Check sheet for the drawn part. Datum: minimum x, y, z corner. Units: mm. A direction names the side the tool comes from. Coordinates: 2 decimals unless noted, no trailing zeros. Order: outer loops, then holes, each group sorted by start corner. A loop starts at its lowest first (then second) coordinate and runs counter-clockwise, first axis right, second up.
Q1. Set-up check for the marked faces 1 and 2: record each of +Z, -Z, +X, -X, +Y, -Y from which the full face is reachable in a straight line by a thin tool's end or side.
Q2. Depth check by flat-ended pin: P1, Ø5, axis at x = 12.5, y = 13.5, coming from the +Z side; P2, Ø2, axis at x = 21, z = 3.5, coming from the +Y side; P3, Ø2, axis at y = 20, z = 11.5, coming from the -X side; P4, Ø5, axis at x = 8, z = 11, coming from the +Y side. Enter the tip coordinate at first touch or a pass-through.
Q3. Cross-section at B-B, the plane z = 7. Record the boundary of the cut face in (x, y), and give its area (3 significant figures).
Q4. Cross-section at A-A, the plane z = 17.75. Record the boundary of the cut face in (x, y), and give its area (3 significant figures).
Q5. Thickness scan on line 1 (X direction, y = 14, z = 17.25); line 2 (X direction, y = 26.5, z = 3). Record the ranges inside material, lowest first.
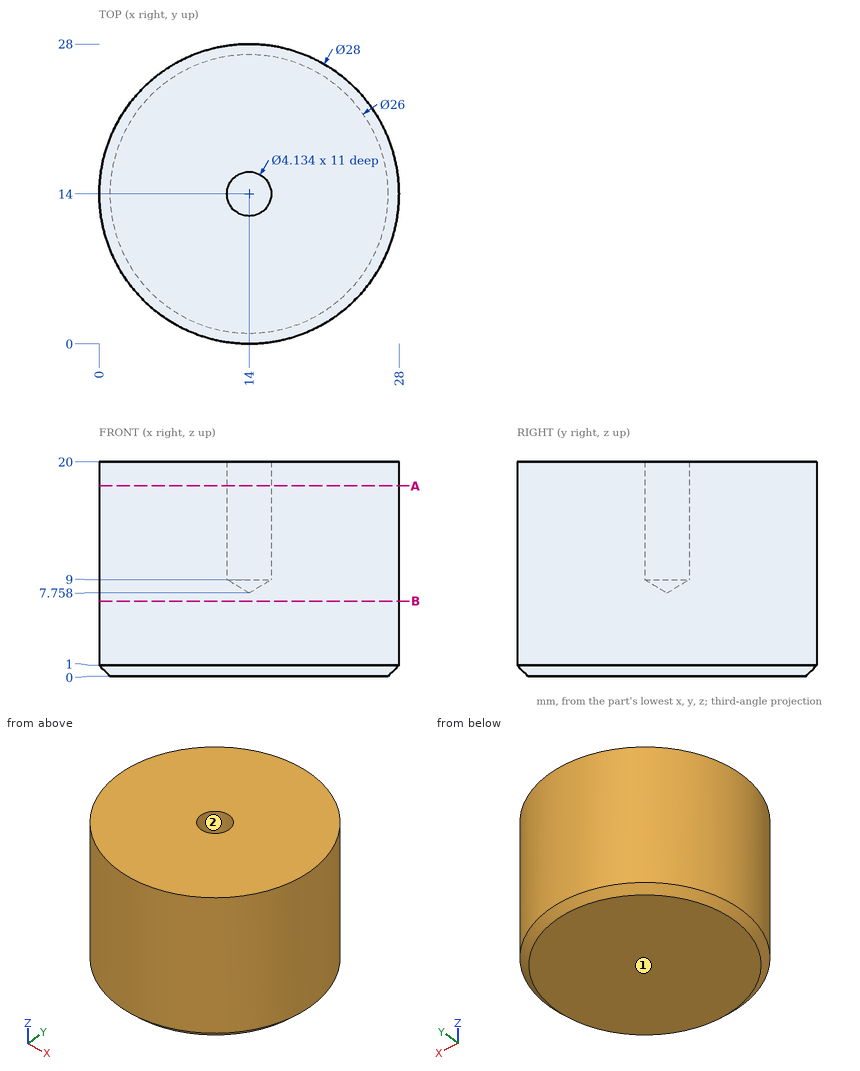
Check values:
1. face 1: -Z, +X, -X, +Y, -Y
1. face 2: +Z
2. P1: stops at z = 20
2. P2: stops at y = 26.65
2. P3: stops at x = 0.92
2. P4: stops at y = 27.56
3. outline: circle Ø28 at (14, 14)
3. area: 616 mm2
4. outline: circle Ø28 at (14, 14); hole circle Ø4.13 at (14, 14)
4. area: 602 mm2
5. line 1: x = 0 to 11.93, 16.07 to 28
5. line 2: x = 7.7 to 20.3
